```python
from build123d import *

# Parameters (mm, degrees)
SKETCH1_R               = 92.71
SKETCH1_R_2             = 53.975
TOP_OF_HATCH_DEPTH      = 3.302
SKETCH2_R               = 92.71
SKETCH2_R_2             = 89.662
HATCH_BODY_DEPTH        = 259.08
SKETCH3_R               = 13.97
CHARGE_TUBE_HOLES_DEPTH = 3.302
SKETCH4_R               = 3.81
BOLT_HOLES_DEPTH        = 263.382
SKETCH_5_R              = 5.08
ANTENNA_HOLES_DEPTH     = 263.382


with BuildPart() as part:
    # Sketch1 → Top of Hatch (new body)
    with BuildSketch(Plane(origin=(0, 0, 0), x_dir=(1, 0, 0), z_dir=(0, 1, 0))):
        Circle(SKETCH1_R)
        Circle(SKETCH1_R_2, mode=Mode.SUBTRACT)
    extrude(amount=TOP_OF_HATCH_DEPTH)

    # Sketch2 → Hatch Body (add)
    with BuildSketch(Plane(origin=(0, 3.302, 0), x_dir=(1, 0, 0), z_dir=(0, 1, 0))):
        Circle(SKETCH2_R)
        Circle(SKETCH2_R_2, mode=Mode.SUBTRACT)
    extrude(amount=HATCH_BODY_DEPTH)

    # Sketch3 → Charge Tube Holes (cut)
    with BuildSketch(Plane.XZ):
        with Locations((-75.565, 0)):
            Circle(SKETCH3_R)
        with Locations((75.565, 0)):
            Circle(SKETCH3_R)
    extrude(amount=-CHARGE_TUBE_HOLES_DEPTH, mode=Mode.SUBTRACT)

    # Sketch4 → Bolt Holes (cut, through all)
    with BuildSketch(Plane.XZ):
        with Locations((38.1, 65.991135768)):
            Circle(SKETCH4_R)
        with Locations((-38.1, 65.991135768)):
            Circle(SKETCH4_R)
        with Locations((-38.1, -65.991135768)):
            Circle(SKETCH4_R)
        with Locations((38.1, -65.991135768)):
            Circle(SKETCH4_R)
    extrude(amount=-BOLT_HOLES_DEPTH, mode=Mode.SUBTRACT)

    # Sketch 5 → Antenna Holes (cut, through all)
    with BuildSketch(Plane.XZ):
        with Locations((-26.112352144, 57.324838678)):
            Circle(SKETCH_5_R)
        with Locations((9.193647856, 61.033450854)):
            Circle(SKETCH_5_R)
    extrude(amount=-ANTENNA_HOLES_DEPTH, mode=Mode.SUBTRACT)


solid = part.part
```
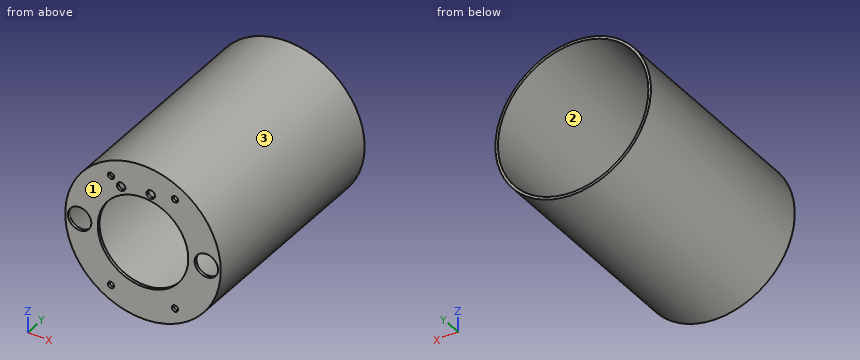
Source: CAD feature listing. Evaluate the final solid. Frame: model axes, mm. Face numbers are marked on the shaded views. Coordinates: 2 decimals unless noted, no trailing zeros. Write each loop counter-clockwise with the first axis right and the second up, starting at its lowest first coordinate (ties: lowest second). Pieces come first, ordered by that corner, then holes. Notation, with made-up numbers: (-18.5, 69.5) - (35.5, 69.5) arc R13 ccw to (35.5, 73.5) - close; hole circle Ø4 at (-37, -5). An arc over 180 degrees is marked (long way). Answer as a JSON object with one key per item and string values.
Q1. Draft query along Z for the marked faces 1, 2 and 3. Return one class per face: released by +Z, released by -Z, zero draft, split by the parting line, or undercut.
Ans:
{"face 1": "zero draft", "face 2": "undercut", "face 3": "split by the parting line"}
Q2. Section query B-B, the plane z = -32.5. Output: boundary loops of the cut face in (x, y).
Ans:
{"outline": "(-86.83, 0) - (-43.09, 0) - (-43.09, 3.3) - (-83.56, 3.3) - (-83.56, 262.38) - (-86.83, 262.38) - close; (43.09, 0) - (86.83, 0) - (86.83, 262.38) - (83.56, 262.38) - (83.56, 3.3) - (43.09, 3.3) - close"}
Q3. Section query C-C, the plane x = -38.1. Output: boundary loops of the cut face in (y, z), plus the area to 3 significant figures.
Ans:
{"outline": "(0, -84.52) - (262.38, -84.52) - (262.38, -81.16) - (3.3, -81.16) - (3.3, -69.8) - (0, -69.8) - close; (0, -62.18) - (3.3, -62.18) - (3.3, -38.23) - (0, -38.23) - close; (0, 38.23) - (3.3, 38.23) - (3.3, 62.18) - (0, 62.18) - close; (0, 69.8) - (3.3, 69.8) - (3.3, 81.16) - (262.38, 81.16) - (262.38, 84.52) - (0, 84.52) - close", "area": "1,990 mm2"}
Q4. Section query A-A, the plane x = 0. Output: boundary loops of the cut face in (y, z) (3 decimals).
Ans:
{"outline": "(0, -92.71) - (262.382, -92.71) - (262.382, -89.662) - (3.302, -89.662) - (3.302, -53.975) - (0, -53.975) - close; (0, 53.975) - (3.302, 53.975) - (3.302, 89.662) - (262.382, 89.662) - (262.382, 92.71) - (0, 92.71) - close"}
Q5. Material intervals for line 1 (Z direction, x = 0, y = 98); line 2 (Y direction, x = 13, z = -77); line 3 (Z direction, x = 38, y = 1), sorted ascending. Write a range as [from, to].
Ans:
{"line 1": "z = [-92.71, -89.66], [89.66, 92.71]", "line 2": "y = [0, 3.3]", "line 3": "z = [-84.56, -69.8], [-62.18, -38.33], [38.33, 62.18], [69.8, 84.56]"}
Q6. Section query D-D, the plane y = 238. Output: boundary loops of the cut face in (x, z), plus the area to 3 significant figures.
Ans:
{"outline": "circle Ø185.42 at (0, 0); hole circle Ø179.32 at (0, 0)", "area": "1,750 mm2"}
Q7. First-contact query: pin 1 Ø4 at (x, y) = (6.5, 48.5) entering from +Z; pin 2 Ø1.5 at (y, z) = (52, -54.5) entering from +X; pin 3 Ø7 at (x, z) = (-38.1, 65.99) entering from +Y; pin 4 Ø2 at (y, z) = (48, 30) entering from +X. Flat tips, straight axial feed; report the tip coordinate or a pass-through.
Ans:
{"pin 1": "stops at z = 92.6", "pin 2": "stops at x = 75.54", "pin 3": "passes through", "pin 4": "stops at x = 88.06"}
